Check sheet for the modelled part. Datum: model origin and axes. Units: mm. Give positions to 0.01 mm unless a question says otherwise; leave off trailing zeros. Write each loop counter-clockwise with the first axis right and the second up, starting at its lowest first coordinate (ties: lowest second). Pieces come first, ordered by that corner, then holes. Notation, with made-up numbers: M 78.25,82.5 L 104.25,82.5 A9 cw 104.25,99.5 Z; hole C 89,-2 d10. An arc over 180 degrees is marked long. Write item = value, one per line. Start each with the question number.
1) Cross-section at A-A, the plane x = 1.75. Record the cut outline in (y, z), plus the area to 3 significant figures.
2) Scan lines: line 1 along Y through (x, z) = (3.75, 0); line 2 along X through (y, z) = (23, -0.25); line 3 along Z through (x, y) = (1.5, 10). Record each from-to range of solid material in increasing order. Write a range as [from, to].
3) Cross-section at C-C, the plane z = -5.75. Record the cut outline in (x, y), plus the area to 3 significant figures.
4) Cross-section at B-B, the plane y = 82.5. Record the cut outline in (x, z), plus the area to 3 significant figures.
5) Go/stop test with flat-tipped pins: pin 1 (3 mm diameter, centred on y = 111, z = -0.5, fed in from -X); pin 2 (1 mm diameter, centred on y = 268, z = 8, fed in from +X); pin 3 (5 mm diameter, centred on y = 32.5, z = -2, fed in from +X); pin 4 (1 mm diameter, centred on x = 3, y = 114.5, fed in from +Z). Record where each tip stops, or that it passes through.
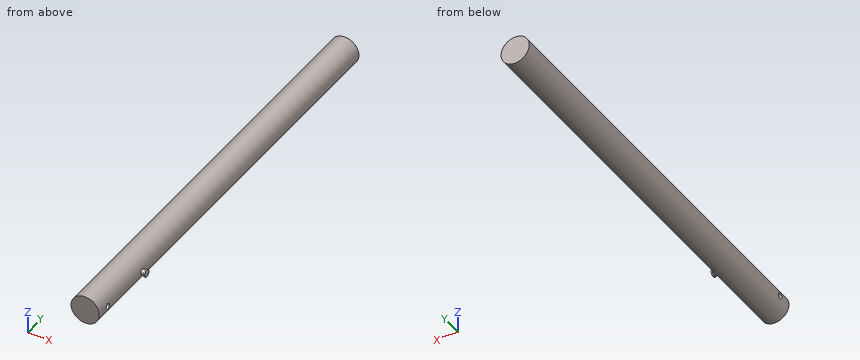
Autodesk Inventor part; units mm, degrees
ref_plane "YZ Plane" through (0, 0, 0) normal (1, 0, 0) x (0, 1, 0)
ref_plane "XZ Plane" through (0, 0, 0) normal (0, 1, 0) x (-1, 0, 0)
ref_plane "XY Plane" through (0, 0, 0) normal (0, 0, 1) x (1, 0, 0)
sketch "Sketch1" plane through (0, 0, 0) normal (0, 1, 0) x (-1, 0, 0)
  circle A0 centre (0, 0) radius 10
  dimension "d0" = 20
extrude "Extrusion1" add sketch "Sketch1" along normal blind 300
sketch "Sketch2" plane through (0, 0, 0) normal (1, 0, 0) x (0, 1, 0)
  circle A0 centre (10, 0) radius 2
  circle A1 centre (50, 0) radius 2
  point P0 (0, 0)
  dimension "d3" = 4
  dimension "d4" = 4
extrude "Extrusion2" cut sketch "Sketch2" along normal mid plane 21 contours A0
sketch "Sketch3" plane through (0, 0, 0) normal (1, 0, 0) x (0, 1, 0)
  circle A0 centre (50, 0) radius 2
  point P0 (0, 0)
  dimension "d7" = 4
extrude "Extrusion3" add sketch "Sketch3" along normal blind 12
sketch "Sketch4" plane through (12, 50, 0) normal (1, 0, 0) x (0, 0, -1)
  circle A0 centre (0, 0) radius 2
  circle A1 centre (0, 0) radius 2.5
  point P0 (0, -50)
  dimension "d10" = 5
extrude "Extrusion4" add sketch "Sketch4" along normal blind 1 contours A0 | A1
properties part number "trail 9"
Reply:
q1.outline = M 0,-9.85 L 300,-9.85 L 300,9.85 L 0,9.85 Z; hole C 10,0 d4
q1.area = 5,890 mm2
q2.line_1 = [0, 8], [12, 300]
q2.line_2 = [-10, 10]
q2.line_3 = [-9.89, -2], [2, 9.89]
q3.outline = M -8.18,0 L 8.18,0 L 8.18,300 L -8.18,300 Z
q3.area = 4,910 mm2
q4.outline = C 0,0 d20
q4.area = 314 mm2
q5.pin_1 = -10
q5.pin_2 = 6.61
q5.pin_3 = 10
q5.pin_4 = 9.68
